Drawing for the job (mm, zero at the part's lowest x, y, z). A direction names the side the tool comes from. Coordinates: 2 decimals unless noted, no trailing zeros. Loops run counter-clockwise (first coordinate to the right, second up) from the corner with the lowest first, then second, coordinate; pieces in that order, holes last. Notation, with made-up numbers: (77.25, 9) - (85.25, 9) arc R24 ccw to (85.25, 46) - close; hole circle Ø8 at (-34.75, 4.25). An arc over 180 degrees is marked (long way). Put each result on its own line as item: value.
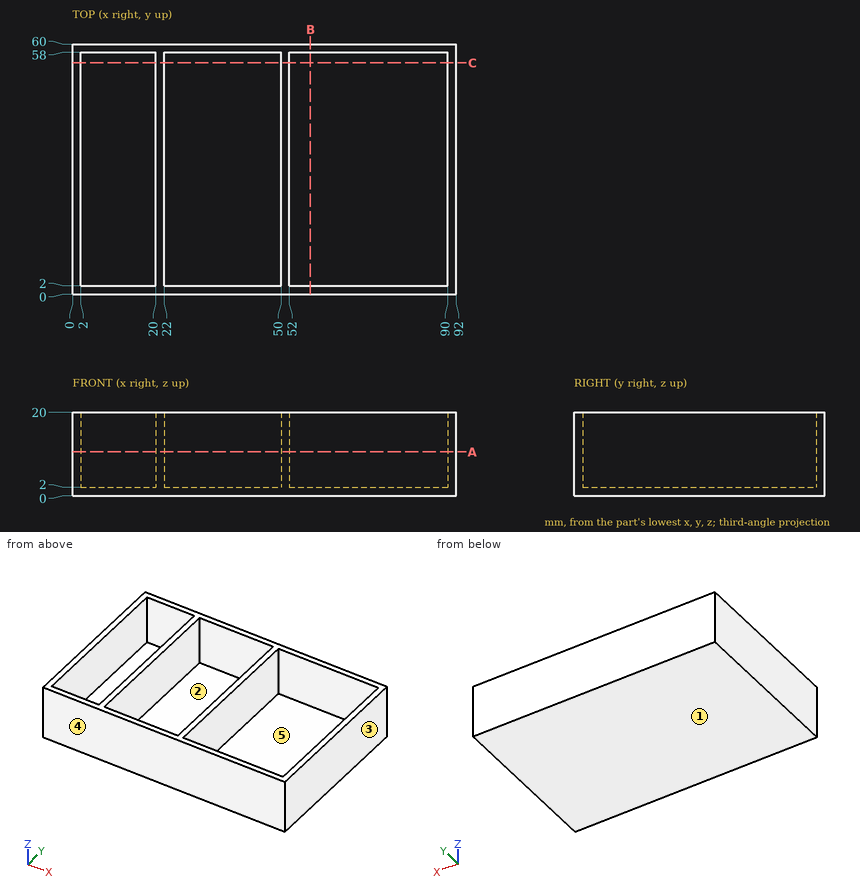
Q1. Slice it at B-B, the plane x = 57. Give the cut face in (y, z), then the cut area to 3 significant figures.
Determined:
outline: (0, 0) - (60, 0) - (60, 20) - (58, 20) - (58, 2) - (2, 2) - (2, 20) - (0, 20) - close
area: 192 mm2
Q2. Mould opens along Y. For the marked faces 3, 4 and 5 say: +Y half, -Y half, draft (parallel to the pull), parting line (faces both ways), or undercut.
Determined:
face 3: draft
face 4: -Y half
face 5: undercut
Q3. Wall check: L1, parallel to X at y = 14, z = 16; L2, parallel to Y at x = 69, z = 14; L3, parallel to Z at x = 78, y = 12. Give the ranges that are in metal, low to high. Write a range as from..to.
Determined:
L1: 0..2, 20..22, 50..52, 90..92
L2: 0..2, 58..60
L3: 0..2
Q4. Slice it at C-C, the plane y = 55.5. Give the cut face in (x, z).
Determined:
outline: (0, 0) - (92, 0) - (92, 20) - (90, 20) - (90, 2) - (52, 2) - (52, 20) - (50, 20) - (50, 2) - (22, 2) - (22, 20) - (20, 20) - (20, 2) - (2, 2) - (2, 20) - (0, 20) - close
Q5. Tool access for the marked faces 1 and 2: list every direction of +Z, -Z, +X, -X, +Y, -Y with a clear straight run to the whole face (end or side of a thin tool).
Determined:
face 1: -Z, +X, -X, +Y, -Y
face 2: +Z
Q6. Pin check, flat tip, straight feed: pin 1 Ø11.5 at (x, y) = (78.5, 30.5) entering from +Z. Stop position of the tip, or through.
Determined:
pin 1: z = 2
Q7. Slice it at A-A, the plane z = 10.5. Give the cut face in (x, y), then the cut area to 3 significant figures.
Determined:
outline: (0, 0) - (92, 0) - (92, 60) - (0, 60) - close; hole (2, 2) - (20, 2) - (20, 58) - (2, 58) - close; hole (22, 2) - (50, 2) - (50, 58) - (22, 58) - close; hole (52, 2) - (90, 2) - (90, 58) - (52, 58) - close
area: 816 mm2
